Can you work these out from the model? Positions are in its coordinate system, mm. A direction names the side the tool comes from. Round coordinates to 2 decimals unless told otherwise and drop trailing zeros. Order: outer loops, then holes, each group sorted by start corner. A loop starts at its lowest first (then second) coordinate and runs counter-clockwise, first axis right, second up. Notation, with made-up numbers: M -38.75,65 L 11.25,65 A29 ccw 11.25,93 Z; hole C 83.25,46 d10. An arc over 180 degrees is marked long. Answer as CSV lines item,"result". Start each with the question number.
from build123d import *

# Parameters (mm, degrees)
BOSS_EXTRUDE1_DEPTH = 11.6
CUT_EXTRUDE1_DEPTH  = 9.85
SKETCH5_W           = 13
SKETCH5_H           = 11.6
CUT_EXTRUDE3_DEPTH  = 51.592094244
CUT_EXTRUDE5_DEPTH  = 9.85
SKETCH9_W           = 29
SKETCH9_H           = 7.5
CUT_EXTRUDE7_DEPTH  = 51.592094244
SKETCH10_R          = 0.75
CUT_EXTRUDE8_DEPTH  = 51.592094244
SKETCH11_W          = 1.5
SKETCH11_H          = 12
CUT_EXTRUDE9_DEPTH  = 10
CUT_EXTRUDE10_DEPTH = 0.75


with BuildPart() as part:
    # Sketch2 → Boss-Extrude1 (new body)
    with BuildSketch(Plane(origin=(0, 0, 0), x_dir=(1, 0, 0), z_dir=(0, 1, 0))):
        Polygon((0, 5.767018283), (0, -6.232981717), (11, -20), (45, -20), (45, 20), (11, 20), align=None)
    extrude(amount=BOSS_EXTRUDE1_DEPTH)

    # Sketch3 → Cut-Extrude1 (cut)
    with BuildSketch(Plane(origin=(0, 11.6, 0), x_dir=(1, 0, 0), z_dir=(0, 1, 0))):
        Polygon((1.5, 7.707879426), (1.5, -8.110302392), (9.5, -18.122679325), (9.5, 18.059138857), align=None)
    extrude(amount=-CUT_EXTRUDE1_DEPTH, mode=Mode.SUBTRACT)

    # Sketch5 → Cut-Extrude3 (cut, through all)
    with BuildSketch(Plane(origin=(0, 11.6, 0), x_dir=(1, 0, 0), z_dir=(0, 1, 0))):
        with Locations((17, 0)):
            Rectangle(SKETCH5_W, SKETCH5_H)
    extrude(amount=-CUT_EXTRUDE3_DEPTH, mode=Mode.SUBTRACT)

    # Sketch7 → Cut-Extrude5 (cut)
    with BuildSketch(Plane(origin=(0, 11.6, 0), x_dir=(1, 0, 0), z_dir=(0, 1, 0))):
        Polygon((1.5, 7.707879426), (0, 5.767018283), (1.5, 5.767018283), align=None)
        Polygon((0, -6.232981717), (1.5, -6.232981717), (1.5, -8.110302392), align=None)
    extrude(amount=-CUT_EXTRUDE5_DEPTH, mode=Mode.SUBTRACT)

    # Sketch9 → Cut-Extrude7 (cut, through all)
    with BuildSketch(Plane.XZ):
        with Locations((30.5, 16.25)):
            Rectangle(SKETCH9_W, SKETCH9_H)
        with Locations((30.5, -16.25)):
            Rectangle(SKETCH9_W, SKETCH9_H)
    extrude(amount=-CUT_EXTRUDE7_DEPTH, mode=Mode.SUBTRACT)

    # Sketch10 → Cut-Extrude8 (cut, through all)
    with BuildSketch(Plane(origin=(0, 11.6, 0), x_dir=(1, 0, 0), z_dir=(0, 1, 0))):
        with Locations(Location((13.5, 16.5, 0), (0, 0, 270))):
            Circle(SKETCH10_R)
        with Locations(Location((13.5, 9, 0), (0, 0, 270))):
            Circle(SKETCH10_R)
        with Locations(Location((41.5, 9, 0), (0, 0, 270))):
            Circle(SKETCH10_R)
        with Locations(Location((41.5, -9.3, 0), (0, 0, 270))):
            Circle(SKETCH10_R)
        with Locations(Location((13.5, -9.3, 0), (0, 0, 270))):
            Circle(SKETCH10_R)
        with Locations(Location((13.5, -16.5, 0), (0, 0, 270))):
            Circle(SKETCH10_R)
    extrude(amount=-CUT_EXTRUDE8_DEPTH, mode=Mode.SUBTRACT)

    # Sketch11 → Cut-Extrude9 (cut)
    with BuildSketch(Plane(origin=(0, 11.6, 0), x_dir=(1, 0, 0), z_dir=(0, 1, 0))):
        Polygon((9.5, 18.059138857), (9.5, -18.122679325), (11, -20), (16, -20), (16, -12.5), (45, -12.5), (45, 12.5), (16, 12.5), (16, 20), (11, 20), align=None)
        with Locations((0.75, -0.232981717)):
            Rectangle(SKETCH11_W, SKETCH11_H)
    extrude(amount=-CUT_EXTRUDE9_DEPTH, mode=Mode.SUBTRACT)

    # Sketch12 → Cut-Extrude10 (cut)
    with BuildSketch(Plane(origin=(0, 1.75, 0), x_dir=(1, 0, 0), z_dir=(0, 1, 0))):
        Polygon((0, 5.767018283), (9.5, 18.059138857), (9.5, -18.122679325), (0, -6.232981717), (1.5, -6.232981717), (1.5, 5.767018283), align=None)
    extrude(amount=-CUT_EXTRUDE10_DEPTH, mode=Mode.SUBTRACT)


solid = part.part
(1) For faces 4 (the flat face through (17, 1, 5.8)), 5 (the flat face through (30, 1, -12.5)), 6 (the flat face through (30, 1, 12.5)), 7 (the flat face through (5.577, 0.611, -12.983)), which set-ups out of +Z, -Z, +X, -X, +Y, -Y let a thin tool reach every point of the face, with its end or its side?
(2) If we mould it in two halves opening along Z, with no side actions, what happens to faces 1 (the flat face through (5.423, 0.611, 13.02)), 2 (the cylindrical face through (42.244, 0.811, -9.098)), 3 (the flat face through (1, 1.6, 0))? For each: +Z half, -Z half, draft (parallel to the pull), parting line (faces both ways), or undercut.
(3) I'm going to push flat-ended pins straight in: P1, Ø1.5, axis at x = 8, z = 10.5, coming from the +Y side; P2, Ø0.8, axis at x = 26.5, y = 0.5, coming from the -Z side. Where does each tip first touch, or does it pass through?
(4) I want a section at B-B on x = 20. Write out the boundary of the cut face in (y, z).
(5) If I drill on line 1 along X through (y, z) = (1.3, -3.5); line 2 along X through (y, z) = (1.25, -9); line 3 along Z through (x, y) = (41.5, 0.4), over which ranges is the centre line in solid material (lowest first)?
(6) I want a section at C-C on z = 9.3. Write out the boundary of the cut face in (x, y), and give its area (3 significant figures).
(7) I want a section at D-D on x = 41.5. Write out the boundary of the cut face in (y, z), and give its area (3 significant figures).
(8) I want a section at A-A on y = 0.45. Write out the boundary of the cut face in (x, z), and give its area (3 significant figures).
From the geometry:
1,face 4,"+Y, -Y"
1,face 5,"-Z, +X, +Y, -Y"
1,face 6,"+Z, +X, +Y, -Y"
1,face 7,"-Z, -X, +Y, -Y"
2,face 1,"+Z half"
2,face 2,"undercut"
2,face 3,"draft"
3,P1,"y = 1"
3,P2,"z = -12.5"
4,outline,"M 0,-12.5 L 1.6,-12.5 L 1.6,-5.8 L 0,-5.8 Z; M 0,5.8 L 1.6,5.8 L 1.6,12.5 L 0,12.5 Z"
5,line 1,"0 to 1.5, 9.5 to 10.5, 23.5 to 45"
5,line 2,"9.5 to 12.75, 14.25 to 40.75, 42.25 to 45"
5,line 3,"-12.5 to -9.75, -8.25 to 8.55, 10.05 to 12.5"
6,outline,"M 2.45,0 L 12.75,0 L 12.75,1.6 L 9.5,1.6 L 9.5,1 L 2.45,1 Z; M 14.25,0 L 40.75,0 L 40.75,1.6 L 14.25,1.6 Z; M 42.25,0 L 45,0 L 45,1.6 L 42.25,1.6 Z"
6,area,"59.0 mm²"
7,outline,"M 0,-12.5 L 1.6,-12.5 L 1.6,-9.75 L 0,-9.75 Z; M 0,-8.25 L 1.6,-8.25 L 1.6,8.55 L 0,8.55 Z; M 0,10.05 L 1.6,10.05 L 1.6,12.5 L 0,12.5 Z"
7,area,"35.2 mm²"
8,outline,"M 0,-5.77 L 11,-20 L 16,-20 L 16,-12.5 L 45,-12.5 L 45,12.5 L 16,12.5 L 16,20 L 11,20 L 0,6.23 Z; hole M 10.5,-5.8 L 23.5,-5.8 L 23.5,5.8 L 10.5,5.8 Z; hole C 13.5,-16.5 d1.5; hole C 13.5,-9 d1.5; hole C 13.5,9.3 d1.5; hole C 13.5,16.5 d1.5; hole C 41.5,-9 d1.5; hole C 41.5,9.3 d1.5"
8,area,"1,050 mm²"
